Autodesk Inventor part; units mm, degrees
ref_plane "YZ Plane" through (0, 0, 0) normal (1, 0, 0) x (0, 1, 0)
ref_plane "XZ Plane" through (0, 0, 0) normal (0, 1, 0) x (-1, 0, 0)
ref_plane "XY Plane" through (0, 0, 0) normal (0, 0, 1) x (1, 0, 0)
sketch "Szkic7" plane through (0, 0, 0) normal (0, 0, 1) x (1, 0, 0)
  circle A0 centre (0, 0) radius 8.331
  dimension "d35" = 16.662
extrude "Wyciągnięcie proste2" add sketch "Szkic7" along normal mid plane 13.275
chamfer "Faza2" distance 1 angle 45 1 edges at (-8.331, 0, 6.6375)
sketch "Szkic9" plane through (0, 0, 6.6375) normal (0, 0, 1) x (1, 0, 0)
  circle A0 centre (0, 0) radius 7.331
extrude "Wyciągnięcie proste3" add sketch "Szkic9" along normal blind 1.125
sketch "Szkic10" plane through (0, 0, 7.7625) normal (0, 0, 1) x (1, 0, 0)
  line L0 (-5.7735, 10) -> (5.7735, 10)
  line L1 (5.7735, 10) -> (11.547, 0)
  line L2 (11.547, 0) -> (5.7735, -10)
  line L3 (5.7735, -10) -> (-5.7735, -10)
  line L4 (-5.7735, -10) -> (-11.547, 0)
  line L5 (-11.547, 0) -> (-5.7735, 10)
  line L6 (0, 11.6634) -> (0, -11.6634) construction
  line L7 (-11.6634, 0) -> (11.6634, 0) construction
  point P0 (0, 0)
  point P1 (0, 0)
  point P2 (0, 10)
  dimension "d44" = 20
extrude "Wyciągnięcie proste4" add sketch "Szkic10" along normal blind 3.6
sketch "Szkic12" plane through (0, 0, 0) normal (0, 1, 0) x (-1, 0, 0)
  line L0 (0, -2.1463) -> (0, 12.8775) construction
  line L1 (-5.7735, 7.7625) -> (-5.7735, 11.3625) construction
  line L2 (-11.547, 11.3625) -> (-5.7735, 11.3625) construction
  line L3 (-11.547, 7.7625) -> (-11.547, 11.3625)
  line L4 (-11.547, 11.0052) -> (-10.2137, 11.3625)
  line L5 (-11.547, 11.3625) -> (-5.7735, 11.3625)
  line L6 (-11.547, 7.7625) -> (-5.7735, 7.7625)
  point P0 (0, 0)
  dimension "d50" = 15
  dimension "d51" = 1.3333
revolve "Obrót2" cut sketch "Szkic12" angle 360 about axis through (0, 0, -10) along (0, 0, 1)
thread "Gwint3"
chamfer "Faza3" distance 1 angle 45 1 edges at (-8.331, 0, -6.6375)
equation "\"d35\" = OD"
equation "\"d36\" = 0.7375 * L"
equation "\"d42\" = 0.0625 * L"
equation "\"d44\" = SW"
equation "\"d45\" = 0.2 * L"
equation "\"d51\" = 0.0666667 * SW"
equation "\"SzerokośćGięciaPodcięcia\" = Grubość"
equation "\"RozmiarPodcięciaNarożnika\" = 4 * Grubość"
equation "\"PromieńPrzejścia\" = PromieńGięcia"
equation "\"Rozmiar_promienia_Jacobiego\" = PromieńGięcia"
equation "\"Wielk_odstępu\" = Grubość"
equation "\"d2\" = PromieńGięcia"
equation "\"d23\" = PromieńGięcia"
equation "\"OD\" = 16.662"
equation "\"SW\" = 20"
equation "\"L\" = 18"
properties part number "Korek sześciokątny BSP 3/8'' L=18" material "304"
Can you work these out from the model? Positions are in its coordinate system, mm. A direction names the side the tool comes from. Give positions to 0.01 mm unless a question says otherwise; leave off trailing zeros. Write each loop counter-clockwise with the first axis right and the second up, starting at its lowest first coordinate (ties: lowest second). Pieces come first, ordered by that corner, then holes. Notation, with made-up numbers: M -11.5,19 L 29.5,19 A13 cw 29.5,39 Z; hole C 20,52 d6. An arc over 180 degrees is marked long. Answer in a Markdown table with one row per item. Add a question column.
Item 1: On a 3-axis mill with a long thin cutter (end or side, diameter ignored), from which of +Z, -Z, +X, -X, +Y, -Y can I reach the whole of each face in a straight line? I mean faces 4 (the conical face through (10.59, 0.05, 11.26)), 5 (the cylindrical face through (-1.81, 8.13, -0.08)), 6 (the flat face through (8, 0, 7.762)). Say none if no direction works.
Item 2: Imagine slicing it at C-C, the plane z = 3.25. Write out the boundary of the cut face in (x, y), plus the area to 3 significant figures.
Item 3: Please list where these lines run through material, in increasing order: L1, parallel to Y at x = 0, z = 5.25; L2, parallel to Z at x = -3.5, y = 8.5.
Item 4: Imagine slicing it at B-B, the plane z = 10.5. Write out the boundary of the cut face in (x, y), plus the area to 3 significant figures.
Item 5: We'd pull the mould along Z, two halves only. Please class faces 1 (the flat face through (8.7, -4.93, 9.54)), 2 (the cylindrical face through (-1.589, 7.157, 7.192)), 3 (the conical face through (-10.59, -0.05, 11.26)): released by +Z, released by -Z, zero draft, split by the parting line, or undercut.
Item 6: For pin 1 Ø3 at (x, z) = (-9, 9.5) entering from +Y; pin 2 Ø4 at (x, z) = (2.5, 1.5) entering from -Y; pin 3 Ø6 at (x, z) = (5.5, -1.5) entering from +Y, each with a flat end and sliding along its axis, tell me the tip position at first contact or that it passes through.
Item 7: Imagine slicing it at A-A, the plane x = 0. Write out the boundary of the cut face in (y, z), plus the area to 3 significant figures.
Evaluation:
| question | item | result |
|---|---|---|
| 1 | face 4 | +Z, +X |
| 1 | face 5 | -Z |
| 1 | face 6 | none |
| 2 | outline | C 0,0 d16.66 |
| 2 | area | 218 mm² |
| 3 | L1 | y = -8.33 to 8.33 |
| 3 | L2 | z = 7.76 to 11.36 |
| 4 | outline | M -11.55,0 L -5.77,-10 L 5.77,-10 L 11.55,0 L 5.77,10 L -5.77,10 Z |
| 4 | area | 346 mm² |
| 5 | face 1 | zero draft |
| 5 | face 2 | undercut |
| 5 | face 3 | released by +Z |
| 6 | pin 1 | stops at y = 7.01 |
| 6 | pin 2 | stops at y = -8.32 |
| 6 | pin 3 | stops at y = 7.95 |
| 7 | outline | M -10,7.76 L -7.33,7.76 L -7.33,6.64 L -8.33,5.64 L -8.33,-5.64 L -7.33,-6.64 L 7.33,-6.64 L 8.33,-5.64 L 8.33,5.64 L 7.33,6.64 L 7.33,7.76 L 10,7.76 L 10,11.36 L -10,11.36 Z |
| 7 | area | 308 mm² |
